Can you work these out from the model? Positions are in its coordinate system, mm. A direction names the side the tool comes from. Coordinates: 2 decimals unless noted, no trailing zeros. Order: outer loops, then holes, each group sorted by start corner. A loop starts at its lowest first (then second) coordinate and runs counter-clockwise, first axis right, second up. Notation, with made-up numbers: (0.5, 3.5) -> (21.5, 3.5) arc R33 ccw to (21.5, 39.5) -> close; hole circle Ø2 at (-32.5, -26.5). An arc over 180 degrees is marked (long way). Use a Markdown table: item, result. Add a question column.
1. For pin 1 Ø5 at (y, z) = (-1.5, 40) entering from +X; pin 2 Ø12 at (x, z) = (30, 26) entering from +Y; pin 3 Ø4 at (x, y) = (40, 9) entering from -Z; pin 4 Ø1.8 at (y, z) = (0.5, 40) entering from +X, each with a flat end and sliding along its axis, tell me the tip position at first contact or that it passes through.
2. If I drill on line 1 along Z through (x, y) = (148, 20.25); line 2 along Y through (x, z) = (89.7, -0.15); line 3 along Z through (x, y) = (27.5, 16.25), over which ranges is the centre line in solid material (lowest first)? Write a range as from..to.
3. We'd pull the mould along Y, two halves only. Please class faces 1 (the flat face through (88.444, 3.217, 21.946)), 2 (the flat face through (179.4, 10, 7)), 3 (the cylindrical face through (170.5, 21.8, 0)), 4 (the flat face through (88.444, 5.074, 23.904)): pulls with the +Y half, pulls with the -Y half, needs draft (parallel to the pull), parting line crosses it, or undercut.
4. For faces 5 (the flat face through (88, 23, 2.5)), 6 (the flat face through (20.4, 0, 36)), 7 (the flat face through (155.4, 0, 36)), which set-ups out of +Z, -Z, +X, -X, +Y, -Y let a thin tool reach every point of the face, with its end or its side?
5. Suppose I cut it at B-B, the plane z = 12.5. List the corners of the cut face in (x, y) for me, then the cut area to 3 significant figures.
6. Suppose I cut it at C-C, the plane z = 23.5. List the corners of the cut face in (x, y) for me.
7. Suppose I cut it at A-A, the plane x = 24. List the corners of the cut face in (y, z) for me, then the cut area to 3 significant figures.
```python
from build123d import *

# Parameters (mm, degrees)
BOSS_EXTRUDE1_DEPTH = 179.4
FILLET1_R           = 10
FILLET3_R           = 2
SKETCH3_R           = 1.55
CUT_EXTRUDE2_DEPTH  = 10
CUT_EXTRUDE4_REACH  = 187.252
SKETCH6_W           = 27
SKETCH6_H           = 20
FILLET4_R           = 2


with BuildPart() as part:
    # Sketch1 → Boss-Extrude1 (new body)
    with BuildSketch(Plane(origin=(0, 0, 0), x_dir=(0, 0, -1), z_dir=(1, 0, 0))):
        Polygon((-2.5, 26.138937515), (-2.5, 12.731613167), (-47.815237798, -3.479647722), (2.5, 9.546261863), (2.5, 26.138937515), align=None)
    extrude(amount=BOSS_EXTRUDE1_DEPTH)

    # Fillet1
    fillet1_edges = [part.edges().sort_by_distance(p)[0] for p in [
        (89.7, 12.731613167, 2.5),
        (89.7, 9.546261863, -2.5),
    ]]
    fillet(fillet1_edges, radius=FILLET1_R)

    # Fillet3
    fillet3_edges = [part.edges().sort_by_distance(p)[0] for p in [
        (89.7, 26.138937515, -2.5),
    ]]
    fillet(fillet3_edges, radius=FILLET3_R)

    # Sketch3 → Cut-Extrude2 (cut, symmetric)
    with BuildSketch(Plane.XY.offset(2.5)):
        with Locations(Location((7.5, 21.138937515, 0), (0, 0, 298.348188053))):
            Circle(SKETCH3_R)
        with Locations(Location((171.9, 21.138937515, 0), (0, 0, 298.348188053))):
            Circle(SKETCH3_R)
        with Locations(Location((89.7, 21.138937515, 0), (0, 0, 298.348188053))):
            Circle(SKETCH3_R)
    extrude(amount=CUT_EXTRUDE2_DEPTH, both=True, mode=Mode.SUBTRACT)

    # Sketch6 → Cut-Extrude4 (cut, up to next)
    with BuildSketch(Plane(origin=(0, 12.079968612, 4.321538013), x_dir=(1, 0, 0), z_dir=(0, 0.9415624549372754, 0.33683845304907145)), mode=Mode.PRIVATE) as cut_extrude4_sk1:
        with Locations((168.9, -36.19311184)):
            Rectangle(SKETCH6_W, SKETCH6_H)
    cut_extrude4_tool1 = extrude(cut_extrude4_sk1.sketch, amount=-CUT_EXTRUDE4_REACH, mode=Mode.PRIVATE) & part.part
    # Sketch6 → Cut-Extrude4 (cut, up to next)
    with BuildSketch(Plane(origin=(0, 12.079968612, 4.321538013), x_dir=(1, 0, 0), z_dir=(0, 0.9415624549372754, 0.33683845304907145)), mode=Mode.PRIVATE) as cut_extrude4_sk2:
        with Locations((123.9, -36.19311184)):
            Rectangle(SKETCH6_W, SKETCH6_H)
    cut_extrude4_tool2 = extrude(cut_extrude4_sk2.sketch, amount=-CUT_EXTRUDE4_REACH, mode=Mode.PRIVATE) & part.part
    # Sketch6 → Cut-Extrude4 (cut, up to next)
    with BuildSketch(Plane(origin=(0, 12.079968612, 4.321538013), x_dir=(1, 0, 0), z_dir=(0, 0.9415624549372754, 0.33683845304907145)), mode=Mode.PRIVATE) as cut_extrude4_sk3:
        with Locations((78.9, -36.19311184)):
            Rectangle(SKETCH6_W, SKETCH6_H)
    cut_extrude4_tool3 = extrude(cut_extrude4_sk3.sketch, amount=-CUT_EXTRUDE4_REACH, mode=Mode.PRIVATE) & part.part
    # Sketch6 → Cut-Extrude4 (cut, up to next)
    with BuildSketch(Plane(origin=(0, 12.079968612, 4.321538013), x_dir=(1, 0, 0), z_dir=(0, 0.9415624549372754, 0.33683845304907145)), mode=Mode.PRIVATE) as cut_extrude4_sk4:
        with Locations((33.9, -36.19311184)):
            Rectangle(SKETCH6_W, SKETCH6_H)
    cut_extrude4_tool4 = extrude(cut_extrude4_sk4.sketch, amount=-CUT_EXTRUDE4_REACH, mode=Mode.PRIVATE) & part.part
    add(cut_extrude4_tool1.solids().sort_by_distance((168.9, -0.111263, 38.399613))[0], mode=Mode.SUBTRACT)
    add(cut_extrude4_tool2.solids().sort_by_distance((123.9, -0.111263, 38.399613))[0], mode=Mode.SUBTRACT)
    add(cut_extrude4_tool3.solids().sort_by_distance((78.9, -0.111263, 38.399613))[0], mode=Mode.SUBTRACT)
    add(cut_extrude4_tool4.solids().sort_by_distance((33.9, -0.111263, 38.399613))[0], mode=Mode.SUBTRACT)

    # Fillet4
    fillet4_edges = [part.edges().sort_by_distance(p)[0] for p in [
        (155.4, 2.405209731, 28.679222311),
        (110.4, 2.405209731, 28.679222311),
        (137.4, 2.405209731, 28.679222311),
        (65.4, 2.405209731, 28.679222311),
        (92.4, 2.405209731, 28.679222311),
        (20.4, 2.405209731, 28.679222311),
        (47.4, 2.405209731, 28.679222311),
    ]]
    fillet(fillet4_edges, radius=FILLET4_R)


solid = part.part
```
Worked out:
| question | item | result |
|---|---|---|
| 1 | pin 1 | stops at x = 155.4 |
| 1 | pin 2 | stops at y = 6.47 |
| 1 | pin 3 | stops at z = -0.28 |
| 1 | pin 4 | passes through |
| 2 | line 1 | z = -2.5..2.5 |
| 2 | line 2 | y = 10.85..19.59, 22.69..26.14 |
| 2 | line 3 | z = -2.45..3.14 |
| 3 | face 1 | pulls with the -Y half |
| 3 | face 2 | needs draft |
| 3 | face 3 | undercut |
| 3 | face 4 | pulls with the +Y half |
| 4 | face 5 | +Z, +X, -X, +Y |
| 4 | face 6 | +Z, +Y, -Y |
| 4 | face 7 | +Z, +X, +Y, -Y |
| 5 | outline | (0, 5.66) -> (179.4, 5.66) -> (179.4, 9.15) -> (0, 9.15) -> close |
| 5 | area | 626 mm² |
| 6 | outline | (0, 2.82) -> (179.4, 2.82) -> (179.4, 5.22) -> (0, 5.22) -> close |
| 7 | outline | (1.55, 28.37) -> (7.61, 4.99) arc R10 ccw to (17.29, -2.5) -> (24.14, -2.5) arc R2 ccw to (26.14, -0.5) -> (26.14, 2.5) -> (19.77, 2.5) arc R10 cw to (10.36, 9.13) -> (3.26, 28.98) -> close |
| 7 | area | 166 mm² |
